Could you check a few things on this model? Use its own coordinates, in mm. A direction names the side the tool comes from. Round coordinates to 2 decimals unless told otherwise and drop trailing zeros. Write each loop counter-clockwise with the first axis right and the second up, starting at its lowest first coordinate (ties: lowest second). Pieces come first, ordered by that corner, then holes. Notation, with made-up numbers: (-22.75, -31) -> (3.25, -31) arc R33 cw to (3.25, 4) -> close; hole circle Ø6 at (-7.5, 80). An arc over 180 degrees is marked (long way). Answer as CSV lines item,"result". Start each with the question number.
Q1. Will these pins go through, and if not, where does the flat tip stop? pin 1 Ø2.5 at (x, z) = (41.5, 3) entering from -Y; pin 2 Ø1.5 at (x, z) = (43, 2) entering from +Y.
Q2. Imagine slicing it at A-A on y = 0. Please give me the cut outline in (x, z).
Q3. If we mould it in two halves opening along X, with no side actions, what happens to faces 1 (the cylindrical face through (-36.688, -53.496, 2.535)), 2 (the flat face through (-22.53, 38.954, 2.465)), 3 (the cylindrical face through (64.673, 5.024, 2.535))? For each: pulls with the +X half, pulls with the -X half, needs draft (parallel to the pull), parting line crosses it, or undercut.
Q4. Imagine slicing it at D-D on z = 3.3. Give the number of separate pieces and of enclosed holes in the cut face, and give its area (3 significant figures).
Q5. Imagine slicing it at C-C on y = 16. Please give me the cut outline in (x, z), and give its area (3 significant figures).
Q6. If I drill on line 1 (X direction, y = -40, z = 4.4); line 2 (Y direction, x = 23, z = 2.8); line 3 (Y direction, x = -28.5, z = 0.2), over which ranges is the centre line in solid material (lowest first)? Write a range as [from, to].
Q7. For faces 4 (the flat face through (20.02, -34.63, 2.46)), 5 (the cylindrical face through (-52.527, -0.758, 2.465)), which set-ups out of +Z, -Z, +X, -X, +Y, -Y let a thin tool reach every point of the face, with its end or its side?
Q8. Imagine slicing it at B-B on x = -10. Please give me the cut outline in (y, z), and give its area (3 significant figures).
from build123d import *

# Parameters (mm, degrees)
ESQUISSE1_R        = 1.65
ESQUISSE1_R_2      = 1.5
ESQUISSE1_W        = 5
ESQUISSE1_H        = 5
BOSS_EXTRU_1_DEPTH = 5
FILLET1_R          = 10


with BuildPart() as part:
    # Esquisse1 → Boss.-Extru.1 (new body)
    with BuildSketch(Plane.XY):
        with BuildLine():
            Line((-36.830127019, 53.791651246), (-28.169872981, 58.791651246))
            ThreePointArc((-28.169872981, 58.791651246), (26.265157649, 45.492587517), (65, 5))
            Line((65, 5), (65, -5))
            ThreePointArc((65, -5), (26.265157649, -45.492587517), (-28.169872981, -58.791651246))
            Line((-28.169872981, -58.791651246), (-36.830127019, -53.791651246))
            ThreePointArc((-36.830127019, -53.791651246), (-52.530315298, 0), (-36.830127019, 53.791651246))
        make_face()
        with Locations((23, 39.837168574)):
            Circle(ESQUISSE1_R, mode=Mode.SUBTRACT)
        with Locations((23, -39.837168574)):
            Circle(ESQUISSE1_R, mode=Mode.SUBTRACT)
        with Locations((-46, 0)):
            Circle(ESQUISSE1_R, mode=Mode.SUBTRACT)
        with Locations((50, 0)):
            Circle(ESQUISSE1_R_2, mode=Mode.SUBTRACT)
        with Locations((-25, 43.301270189)):
            Circle(ESQUISSE1_R_2, mode=Mode.SUBTRACT)
        with Locations((-25, -43.301270189)):
            Circle(ESQUISSE1_R_2, mode=Mode.SUBTRACT)
        with BuildLine():
            Line((15.669872981, 37.141016151), (24.330127019, 32.141016151))
            ThreePointArc((24.330127019, 32.141016151), (32.145280949, 0), (24.330127019, -32.141016151))
            Line((24.330127019, -32.141016151), (15.669872981, -37.141016151))
            ThreePointArc((15.669872981, -37.141016151), (-16.072640474, -27.838629914), (-40, -5))
            Line((-40, -5), (-40, 5))
            ThreePointArc((-40, 5), (-16.072640474, 27.838629914), (15.669872981, 37.141016151))
        make_face(mode=Mode.SUBTRACT)
        with Locations((42.5, 0)):
            Rectangle(ESQUISSE1_W, ESQUISSE1_H, mode=Mode.SUBTRACT)
        with Locations((57.5, 0)):
            Rectangle(ESQUISSE1_W, ESQUISSE1_H, mode=Mode.SUBTRACT)
        Polygon((-25.334936491, 48.881397208), (-27.834936491, 53.211524227), (-32.165063509, 50.711524227), (-29.665063509, 46.381397208), align=None, mode=Mode.SUBTRACT)
        Polygon((-20.334936491, 40.22114317), (-17.834936491, 35.891016151), (-22.165063509, 33.391016151), (-24.665063509, 37.72114317), align=None, mode=Mode.SUBTRACT)
        Polygon((-29.665063509, -46.381397208), (-32.165063509, -50.711524227), (-27.834936491, -53.211524227), (-25.334936491, -48.881397208), align=None, mode=Mode.SUBTRACT)
        Polygon((-24.665063509, -37.72114317), (-22.165063509, -33.391016151), (-17.834936491, -35.891016151), (-20.334936491, -40.22114317), align=None, mode=Mode.SUBTRACT)
    extrude(amount=BOSS_EXTRU_1_DEPTH)

    # Fillet1
    fillet1_edges = [part.edges().sort_by_distance(p)[0] for p in [
        (-36.830127019, 53.791651246, 2.5),
        (-28.169872981, 58.791651246, 2.5),
        (65, 5, 2.5),
        (65, -5, 2.5),
        (-28.169872981, -58.791651246, 2.5),
        (-36.830127019, -53.791651246, 2.5),
        (15.669872981, 37.141016151, 2.5),
        (-40, 5, 2.5),
        (-40, -5, 2.5),
        (15.669872981, -37.141016151, 2.5),
        (24.330127019, -32.141016151, 2.5),
        (24.330127019, 32.141016151, 2.5),
    ]]
    fillet(fillet1_edges, radius=FILLET1_R)


solid = part.part
Checks:
1,pin 1,"y = -35.74"
1,pin 2,"y = 34.03"
2,outline,"(-52.53, 0) -> (-47.65, 0) -> (-47.65, 5) -> (-52.53, 5) -> close; (-44.35, 0) -> (-40, 0) -> (-40, 5) -> (-44.35, 5) -> close; (32.15, 0) -> (40, 0) -> (40, 5) -> (32.15, 5) -> close; (45, 0) -> (48.5, 0) -> (48.5, 5) -> (45, 5) -> close; (51.5, 0) -> (55, 0) -> (55, 5) -> (51.5, 5) -> close; (60, 0) -> (65, 0) -> (65, 5) -> (60, 5) -> close"
3,face 1,"pulls with the -X half"
3,face 2,"undercut"
3,face 3,"pulls with the +X half"
4,separate pieces,"1"
4,enclosed holes,"13"
4,area,"6,200 mm^2"
5,outline,"(-51.24, 0) -> (-31.27, 0) -> (-31.27, 5) -> (-51.24, 5) -> close; (30.29, 0) -> (58.35, 0) -> (58.35, 5) -> (30.29, 5) -> close"
5,area,"240 mm^2"
6,line 1,"[-44.18, -20.72], [-20.21, 21.36], [24.64, 34.76]"
6,line 2,"[-47.3, -41.49], [-38.19, -32.76], [32.76, 38.19], [41.49, 47.3]"
6,line 3,"[-58.36, -52.83], [-47.05, -18.7], [18.7, 47.05], [52.83, 58.36]"
7,face 4,"+Z, -Z"
7,face 5,"+Z, -Z, -X"
8,outline,"(-57.94, 0) -> (-30.96, 0) -> (-30.96, 5) -> (-57.94, 5) -> close; (30.96, 0) -> (57.94, 0) -> (57.94, 5) -> (30.96, 5) -> close"
8,area,"270 mm^2"
